```python
from build123d import *

# Parameters (mm, degrees)
DODANIE_WYCI_GNI_CIE1_DEPTH = 342
SZKIC3_W                    = 2
SZKIC3_H                    = 15
DODANIE_WYCI_GNI_CIE2_DEPTH = 12
SZKIC4_R                    = 2
WYTNIJ_WYCI_GNI_CIE1_DEPTH  = 10
SZKIC5_R                    = 2
WYTNIJ_WYCI_GNI_CIE2_DEPTH  = 10


with BuildPart() as part:
    # Szkic1 → Dodanie-wyciągnięcie1 (new body)
    with BuildSketch(Plane(origin=(0, 0, 0), x_dir=(1, 0, 0), z_dir=(0, 1, 0))):
        Polygon((0, 0), (0, 2), (32, 2), (32, 32), (32.5, 32), (32.5, 2.5), (42, 2.5), (42, 2), (68, 2), (68, 0), align=None)
    extrude(amount=DODANIE_WYCI_GNI_CIE1_DEPTH)

    # Szkic3 → Dodanie-wyciągnięcie2 (add)
    with BuildSketch(Plane(origin=(0, 0, -2), x_dir=(-1, 0, 0), z_dir=(0, 0, -1))):
        with Locations((-67, 82.5)):
            Rectangle(SZKIC3_W, SZKIC3_H)
        with Locations((-67, 259.5)):
            Rectangle(SZKIC3_W, SZKIC3_H)
        with Locations((-1, 82.5)):
            Rectangle(SZKIC3_W, SZKIC3_H)
        with Locations((-1, 259.5)):
            Rectangle(SZKIC3_W, SZKIC3_H)
    extrude(amount=DODANIE_WYCI_GNI_CIE2_DEPTH)

    # Szkic4 → Wytnij-wyciągnięcie1 (cut)
    with BuildSketch(Plane.ZY):
        with Locations((-9, 82.5)):
            Circle(SZKIC4_R)
        with Locations((-9, 259.5)):
            Circle(SZKIC4_R)
    extrude(amount=-WYTNIJ_WYCI_GNI_CIE1_DEPTH, mode=Mode.SUBTRACT)

    # Szkic5 → Wytnij-wyciągnięcie2 (cut)
    with BuildSketch(Plane(origin=(68, 0, 0), x_dir=(0, 0, -1), z_dir=(1, 0, 0))):
        with Locations((9, 259.5)):
            Circle(SZKIC5_R)
        with Locations((9, 82.5)):
            Circle(SZKIC5_R)
    extrude(amount=-WYTNIJ_WYCI_GNI_CIE2_DEPTH, mode=Mode.SUBTRACT)


solid = part.part
```
For this review, take the finished solid that the model builds, in its own axes (mm). A direction names the side the tool comes from. Round coordinates to 2 decimals unless told otherwise and drop trailing zeros. Write each loop counter-clockwise with the first axis right and the second up, starting at its lowest first coordinate (ties: lowest second). Pieces come first, ordered by that corner, then holes.
1) Take a section at A-A on y = 185.5. Give the boundary of the cut face in (x, z).
Answer below:
outline: (0, -2) - (32, -2) - (32, -32) - (32.5, -32) - (32.5, -2.5) - (42, -2.5) - (42, -2) - (68, -2) - (68, 0) - (0, 0) - close
2) Machinability: for faces 4 (the face through (68, 170.2, -1.8)), 5 (the face through (2, 82.4, -6.6)), which of the approach directions +Z, -Z, +X, -X, +Y, -Y give a long, thin tool a straight path to every point of the face, cutting with its end or side? Answer none if there is none.
Answer below:
face 4: +Z, -Z, +X, +Y, -Y
face 5: -Z, +Y, -Y
3) Insertion check: pin 1 Ø2 at (x, z) = (1, -5.5) entering from -Y; pin 2 Ø6 at (x, y) = (49, 147) entering from -Z; pin 3 Ø2 at (y, z) = (134, -10.5) entering from -X. Each pin has a flat end and moves straight along its axis. Give the tip position at first contact, or say it passes through.
Answer below:
pin 1: stops at y = 75
pin 2: stops at z = -2
pin 3: stops at x = 32
4) Take a section at B-B on x = 36.5. Give the boundary of the cut face in (y, z), then the cut area to 3 significant figures.
Answer below:
outline: (0, -2.5) - (342, -2.5) - (342, 0) - (0, 0) - close
area: 855 mm2
5) Mouldability with a two-part tool opening along X and no side actions: class faces 1 (the face through (2, 259.4, -6.6)), 2 (the face through (0, 170, -1)), 3 (the face through (34, 342, -2)) as +X half, -X half, draft (parallel to the pull), parting line (faces both ways), or undercut.
Answer below:
face 1: undercut
face 2: -X half
face 3: draft
6) For line 1 along Y through (x, z) = (0.65, -9); line 2 along X through (y, z) = (226, -21); line 3 along Z through (x, y) = (67, 82), list the stretches that pass through material, from the lowest coordinate up.
Answer below:
line 1: y = 75 to 80.5, 84.5 to 90, 252 to 257.5, 261.5 to 267
line 2: x = 32 to 32.5
line 3: z = -14 to -10.94, -7.06 to 0
7) Take a section at C-C on z = -24.5. Give the boundary of the cut face in (x, y), then the cut area to 3 significant figures.
Answer below:
outline: (32, 0) - (32.5, 0) - (32.5, 342) - (32, 342) - close
area: 171 mm2
